CAD build for the part. Positions are in the model's coordinates, mm. A direction names the side the tool comes from. Give positions to 0.01 mm unless a question says otherwise; leave off trailing zeros. Write each loop counter-clockwise with the first axis right and the second up, starting at its lowest first coordinate (ties: lowest second). Pieces come first, ordered by that corner, then holes. Notation, with made-up numbers: (-1.75, 62) -> (7.25, 62) arc R15 ccw to (7.25, 75) -> close; hole circle Ø9 at (73, 10.5). An arc over 180 degrees is marked (long way). Answer in a Markdown table with one row per item. Add a question column.
```python
from build123d import *

# Parameters (mm, degrees)
SKETCH1_W      = 2
SKETCH1_H      = 40
MAIN_ANGLE     = 90
SUPPORT_DEPTH  = 10
SKETCH6_W      = 1
SKETCH6_H      = 2.9
FIX_2_DEPTH    = 10
SKETCH9_R      = 1.6
HOLES_DEPTH    = 5
SKETCH10_R     = 4.5
BIGHOLES_DEPTH = 17.5


with BuildPart() as part:
    # Sketch1 → Main (revolve, symmetric)
    with BuildSketch(Plane.XY) as main_sk:
        with Locations((48.5, 20)):
            Rectangle(SKETCH1_W, SKETCH1_H)
    revolve(axis=Axis((0, -0.284703924, 0), (0, 1, 0)), revolution_arc=MAIN_ANGLE / 2)
    revolve(main_sk.sketch, axis=Axis((0, -0.284703924, 0), (0, -1, 0)), revolution_arc=MAIN_ANGLE / 2)

    # Sketch2 → Support (add)
    with BuildSketch(Plane(origin=(0, 10, 0), x_dir=(-1, 0, 0), z_dir=(0, -1, 0))):
        with BuildLine():
            Line((-47.236109069, -5), (-33, -5))
            Line((-33, -5), (-33, 5))
            Line((-33, 5), (-47.236109069, 5))
            ThreePointArc((-47.236109069, 5), (-46.422799712, 10.058512159), (-45.069390943, 15))
            Line((-45.069390943, 15), (-30, 15))
            Line((-30, 15), (-30, -15))
            Line((-30, -15), (-45.069390943, -15))
            ThreePointArc((-45.069390943, -15), (-46.422799712, -10.058512159), (-47.236109069, -5))
        make_face()
    extrude(amount=-SUPPORT_DEPTH)

    # Sketch6 → Fix 2 (add)
    with BuildSketch(Plane(origin=(0, 10, 0), x_dir=(1, 0, 0), z_dir=(0, 1, 0))):
        with Locations((29.5, -10)):
            Rectangle(SKETCH6_W, SKETCH6_H)
        with Locations((29.5, 10)):
            Rectangle(SKETCH6_W, SKETCH6_H)
    extrude(amount=FIX_2_DEPTH)

    # Sketch9 → Holes (cut, through all)
    with BuildSketch(Plane(origin=(33, 0, 0), x_dir=(0, 0, -1), z_dir=(1, 0, 0))):
        with Locations((10, 15)):
            Circle(SKETCH9_R)
        with Locations((-10, 15)):
            Circle(SKETCH9_R)
    extrude(amount=-HOLES_DEPTH, mode=Mode.SUBTRACT)

    # Sketch10 → BigHoles (cut, through all)
    with BuildSketch(Plane(origin=(33, 0, 0), x_dir=(0, 0, -1), z_dir=(1, 0, 0))):
        with Locations((10, 15)):
            Circle(SKETCH10_R)
        with Locations((-10, 15)):
            Circle(SKETCH10_R)
    extrude(amount=BIGHOLES_DEPTH, mode=Mode.SUBTRACT)


solid = part.part
```
Item 1: Slice it at C-C, the plane y = 15. List the corners of the cut face in (x, z).
Item 2: Probe L1, parallel to Y at x = 31.45, z = 10; L2, parallel to Z at x = 37, y = 15; L3, parallel to Z at x = 44, y = 15. List the from-to ranges inside material, lowest first. Write a range as from..to.
Item 3: Slice it at B-B, the plane x = 36. List the corners of the cut face in (y, z).
Item 4: Mould opens along X. For faces 5 (the face through (33, 15, 0)), 6 (the face through (40.983, 16.352, 5.708)), 7 (the face through (40, 15, -5)), 8 (the face through (33, 13, -10)) say: released by +X, released by -X, zero draft, split by the parting line, or undercut.
Item 5: Which spindle directions (+Z, -Z, +X, -X, +Y, -Y) get a long thin tool onto all of the face, cutting with end or side? Do faces 1 (the face through (32, 10, 0)), 2 (the face through (33, 13, 10)), 3 (the face through (32, 20, 0)), 4 (the face through (30, 15, 13)). Say none if no direction does.
Item 6: Drop flat-ended pins along their axis: pin 1 Ø3 at (y, z) = (25, -18) entering from -X; pin 2 Ø10 at (y, z) = (14, 10.5) entering from +X; pin 3 Ø6 at (y, z) = (14.5, -3.5) entering from -X; pin 4 Ø1.9 at (y, z) = (15, -10) entering from -X. Give the stop position or say it passes through.
Item 7: Slice it at A-A, the plane z = 2.5. List the corners of the cut face in (x, y).
Item 8: Slice it at D-D, the plane x = 39.5. List the corners of the cut face in (y, z).
Answer key:
| question | item | result |
|---|---|---|
| 1 | outline | (30, -15) -> (45.07, -15) arc R47.5 cw to (33.59, -33.59) -> (35, -35) arc R49.5 ccw to (47.33, -14.5) -> (33, -14.5) -> (33, -11.6) -> (30, -11.6) -> close; (30, -8.4) -> (33, -8.4) -> (33, -5.5) -> (49.19, -5.5) arc R49.5 ccw to (49.19, 5.5) -> (33, 5.5) -> (33, 8.4) -> (30, 8.4) -> close; (30, 11.6) -> (33, 11.6) -> (33, 14.5) -> (47.33, 14.5) arc R49.5 ccw to (35, 35) -> (33.59, 33.59) arc R47.5 cw to (45.07, 15) -> (30, 15) -> close; hole (33, -5) -> (47.24, -5) arc R47.5 ccw to (47.24, 5) -> (33, 5) -> close |
| 2 | L1 | y = 10..13.4, 16.6..20 |
| 2 | L2 | z = -32.88..-29.79, -15..-14.5, -5.5..-5, 5..5.5, 14.5..15, 29.79..32.88 |
| 2 | L3 | z = -22.68..-17.9, -15..-14.5, -5.5..-5, 5..5.5, 14.5..15, 17.9..22.68 |
| 3 | outline | (0, -33.97) -> (40, -33.97) -> (40, -30.99) -> (0, -30.99) -> close; (0, 30.99) -> (40, 30.99) -> (40, 33.97) -> (0, 33.97) -> close; (10, -15) -> (20, -15) -> (20, -5) -> (10, -5) -> close; (10, 5) -> (20, 5) -> (20, 15) -> (10, 15) -> close; hole circle Ø9 at (15, -10); hole circle Ø9 at (15, 10) |
| 4 | face 5 | undercut |
| 4 | face 6 | zero draft |
| 4 | face 7 | undercut |
| 4 | face 8 | released by +X |
| 5 | face 1 | -X, -Y |
| 5 | face 2 | +X |
| 5 | face 3 | -X, +Y |
| 5 | face 4 | +Z, -X, +Y, -Y |
| 6 | pin 1 | stops at x = 43.31 |
| 6 | pin 2 | stops at x = 49.19 |
| 6 | pin 3 | stops at x = 30 |
| 6 | pin 4 | passes through |
| 7 | outline | (30, 10) -> (33, 10) -> (33, 20) -> (30, 20) -> close; (47.43, 0) -> (49.44, 0) -> (49.44, 40) -> (47.43, 40) -> close |
| 8 | outline | (0, -29.83) -> (40, -29.83) -> (40, -26.38) -> (0, -26.38) -> close; (0, 26.38) -> (40, 26.38) -> (40, 29.83) -> (0, 29.83) -> close; (10, -15) -> (20, -15) -> (20, -5) -> (10, -5) -> close; (10, 5) -> (20, 5) -> (20, 15) -> (10, 15) -> close; hole circle Ø9 at (15, -10); hole circle Ø9 at (15, 10) |
